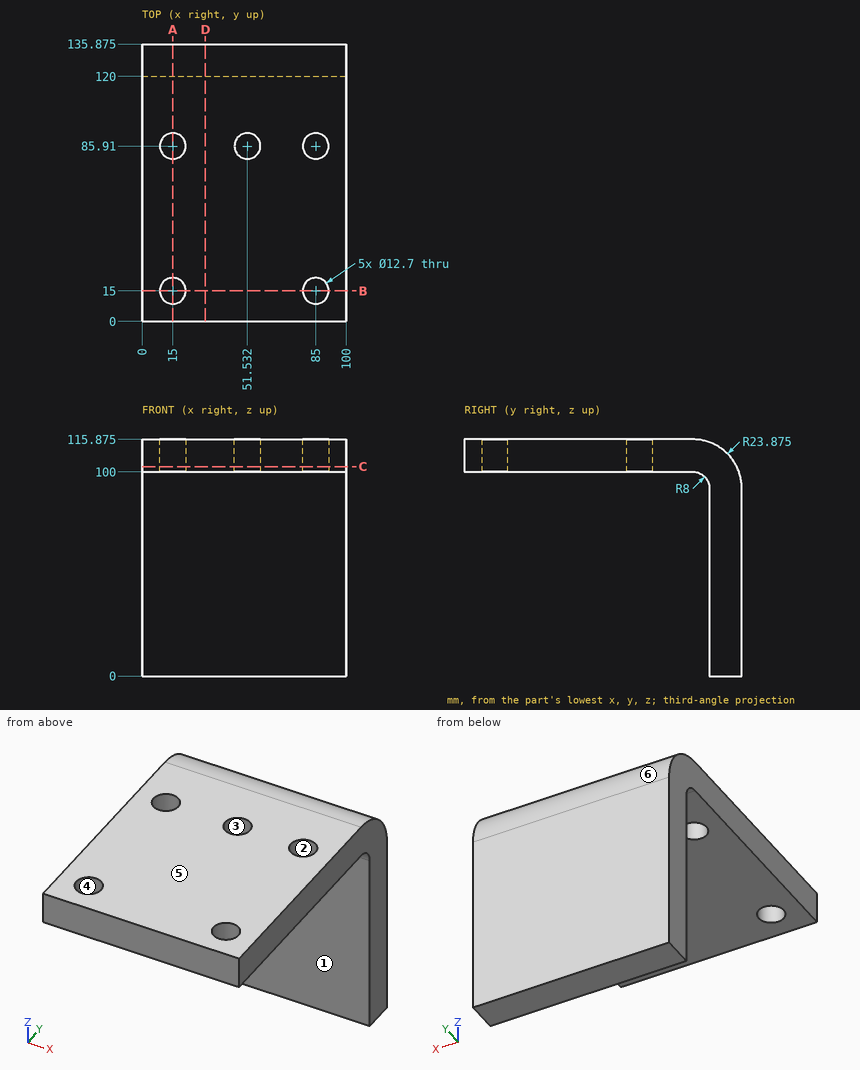
Could you check a few things on this drawing? It's one solid part, dimensions in mm from its lowest x, y, z. A direction names the side the tool comes from. Round coordinates to 2 decimals unless told otherwise and drop trailing zeros. Write each loop counter-clockwise with the first axis right and the second up, starting at its lowest first coordinate (ties: lowest second). Pieces come first, ordered by that corner, then holes.
Q1. If we section it at B-B on y = 15: Write out the boundary of the cut face in (x, z) (3 decimals).
Q2. Please list where these lines run through material, in increasing order: probe 1 along Y at (x, z) = (15, 106.5); probe 2 along Y at (x, z) = (85, 111); probe 3 along Y at (x, z) = (70.5, 23) (3 decimals).
Q3. Will these pins go through, and if not, where does the flat tip stop? P1, Ø8, axis at x = 17.5, y = 33, coming from the -Z side; P2, Ø3, axis at x = 10, z = 48.5, coming from the -Y side.
Q4. If we section it at C-C on z = 102.5: Write out the boundary of the cut face in (x, y), plus the area to 3 significant figures.
Q5. Which directions (+Z, -Z, +X, -X, +Y, -Y) give clear straight access to the entire face, cutting with the end or side of a thin tool? Please do the marked faces 1 and 2.
Q6. If we mould it in two halves opening along Y, with no side actions, what happens to the marked faces 3, 4, 5 and 6? For each: +Y half, -Y half, draft (parallel to the pull), parting line (faces both ways), or undercut.
Q7. If we section it at A-A on x = 15: Write out the boundary of the cut face in (y, z) (3 decimals).
Q8. If we section it at D-D on x = 31: Write out the boundary of the cut face in (y, z) (3 decimals), plus the area to 3 significant figures.
Answer below:
1. outline: (0, 100) - (8.65, 100) - (8.65, 115.875) - (0, 115.875) - close; (21.35, 100) - (78.65, 100) - (78.65, 115.875) - (21.35, 115.875) - close; (91.35, 100) - (100, 100) - (100, 115.875) - (91.35, 115.875) - close
2. probe 1: y = 0 to 8.65, 21.35 to 79.56, 92.26 to 130.97
2. probe 2: y = 0 to 8.65, 21.35 to 79.56, 92.26 to 126.46
2. probe 3: y = 120 to 135.875
3. P1: stops at z = 100
3. P2: stops at y = 120
4. outline: (0, 0) - (100, 0) - (100, 133.44) - (0, 133.44) - close; hole circle Ø12.7 at (15, 15); hole circle Ø12.7 at (15, 85.91); hole circle Ø12.7 at (51.53, 85.91); hole circle Ø12.7 at (85, 15); hole circle Ø12.7 at (85, 85.91)
4. area: 12,700 mm2
5. face 1: -Z, +X, -X, -Y
5. face 2: +Z, -Z
6. face 3: undercut
6. face 4: undercut
6. face 5: draft
6. face 6: +Y half
7. outline: (0, 100) - (8.65, 100) - (8.65, 115.875) - (0, 115.875) - close; (21.35, 100) - (79.56, 100) - (79.56, 115.875) - (21.35, 115.875) - close; (92.26, 100) - (112, 100) arc R8 cw to (120, 92) - (120, 0) - (135.875, 0) - (135.875, 92) arc R23.875 ccw to (112, 115.875) - (92.26, 115.875) - close
8. outline: (0, 100) - (112, 100) arc R8 cw to (120, 92) - (120, 0) - (135.875, 0) - (135.875, 92) arc R23.875 ccw to (112, 115.875) - (0, 115.875) - close
8. area: 3,640 mm2
